```python
from build123d import *

# Parameters (mm, degrees)
SKETCH2_R          = 24
SKETCH2_R_2        = 10.5
CUT_EXTRUDE1_DEPTH = 2
FILLET1_R          = 1


with BuildPart() as part:
    # Sketch1 → Revolve1 (revolve)
    with BuildSketch(Plane.XY, mode=Mode.PRIVATE) as revolve1_sk:
        Polygon((-3.5, 6), (-3.5, 0), (-30, 0), (-28.5, 1.5), (-30, 3), (-7.5, 3), (-6, 4.5), (-7.5, 6), align=None)
    revolve(revolve1_sk.sketch.rotate(Axis((0, 0, 0), (0, 1, 0)), 270), axis=Axis((0, 0, 0), (0, 1, 0)))

    # Sketch2 → Cut-Extrude1 (cut)
    with BuildSketch(Plane(origin=(0, 3, 0), x_dir=(1, 0, 0), z_dir=(0, 1, 0))):
        with Locations(Location((0, 0, 0), (0, 0, 270))):
            Circle(SKETCH2_R)
        with Locations(Location((0, 0, 0), (0, 0, 270))):
            Circle(SKETCH2_R_2, mode=Mode.SUBTRACT)
    extrude(amount=-CUT_EXTRUDE1_DEPTH, mode=Mode.SUBTRACT)

    # Fillet1
    fillet1_edges = [part.edges().sort_by_distance(p)[0] for p in [
        (0, 1, -10.5),
        (0, 1, -24),
    ]]
    fillet(fillet1_edges, radius=FILLET1_R)
    fillet1_2_edges = [part.edges().sort_by_distance(p)[0] for p in [
        (0, 3, -24),
        (0, 3, -10.5),
    ]]
    fillet(fillet1_2_edges, radius=FILLET1_R - 0.0001)  # a hair under: the kernel refuses the full size


solid = part.part
```
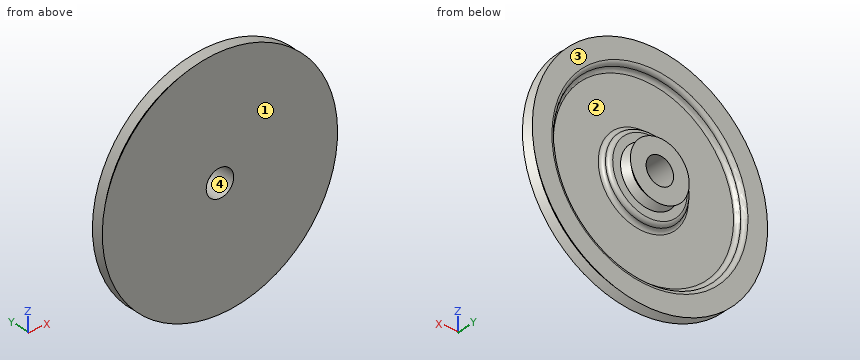
Geometry check sheet. Reference: the model listing, model coordinates, mm. Face numbers are marked on the shaded views. A direction names the side the tool comes from. Round coordinates to 2 decimals unless told otherwise and drop trailing zeros. Use a Markdown table: item, result.
(1) Set-up check for the marked faces 1 and 2: record each of +Z, -Z, +X, -X, +Y, -Y from which the full face is reachable in a straight line by a thin tool's end or side.
Calculated:
| item | result |
|---|---|
| face 1 | +Z, -Z, +X, -X, -Y |
| face 2 | +Y |
(2) Scan lines: probe 1 along X at (y, z) = (1.7, 0); probe 2 along X at (y, z) = (2.05, 0); probe 3 along Y at (x, z) = (8, 10). Record each from-to range of solid material in increasing order.
Calculated:
| item | result |
|---|---|
| probe 1 | -28.7 to -23.95, -10.55 to -3.5, 3.5 to 10.55, 23.95 to 28.7 |
| probe 2 | -29.05 to -24, -10.5 to -3.5, 3.5 to 10.5, 24 to 29.05 |
| probe 3 | 0 to 1 |
(3) Go/stop test with flat-tipped pins: P1, Ø1.5, axis at y = 4, z = -6, coming from the -X side; P2, Ø1.5, axis at x = 6.5, z = 23.5, coming from the +Y side; P3, Ø3, axis at y = 0.5, z = -19.5, coming from the +X side. Record where each tip stops, or that it passes through.
Calculated:
| item | result |
|---|---|
| P1 | x = -4.43 |
| P2 | y = 3 |
| P3 | x = 23.94 |
(4) Mould release check, pull along Z, two halves, no side actions. Record for the marked faces 3 and 4: released by +Z, released by -Z, zero draft, split by the parting line, or undercut.
Calculated:
| item | result |
|---|---|
| face 3 | zero draft |
| face 4 | undercut |
